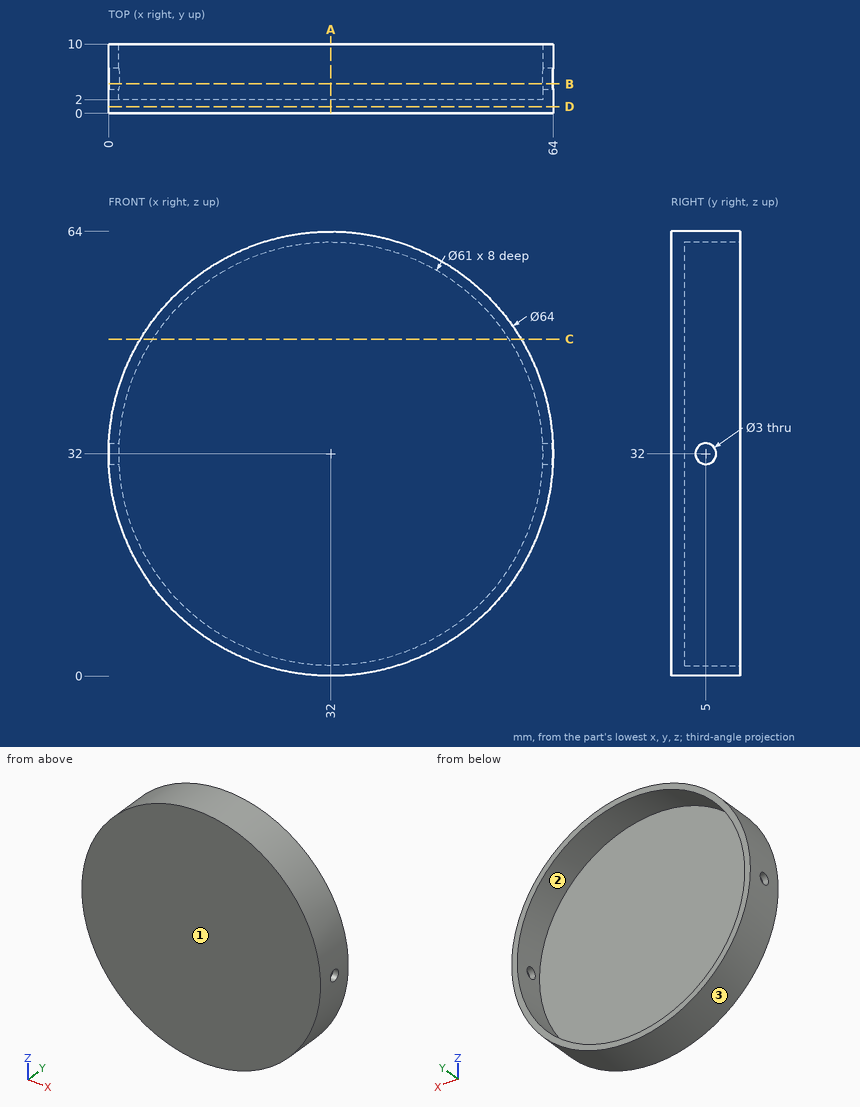
The drawing under review shows one solid part. Ordinate dimensions are in mm from its lowest x, y, z. Give positions to 0.01 mm unless a question says otherwise; leave off trailing zeros. Order: outer loops, then holes, each group sorted by start corner. A loop starts at its lowest first (then second) coordinate and runs counter-clockwise, first axis right, second up. Notation, with made-up numbers: M 4.5,28 L 26.5,28 A18 cw 26.5,52 Z; hole C 72,42 d2. An arc over 180 degrees is marked long. Answer in a Markdown table with one row per item. Add a question column.
1. Add section A-A on x = 32. State the section outline as (y, z) points, plus the area to 3 significant figures.
2. Add section B-B on y = 4.25. State the section outline as (x, z) points.
3. Add section C-C on z = 48.5. State the section outline as (x, y) points.
4. Add section D-D on y = 1. State the section outline as (x, z) points, plus the area to 3 significant figures.
5. To check wall thickness, follow line 1 along Z through (x, y) = (32, 8.5); line 2 along Y through (x, z) = (17.5, 58); line 3 along Z through (x, y) = (35, 5.75). State the ranges of each line that lie inside material, in increasing order.
6. For pin 1 Ø2 at (x, z) = (32.5, 27) entering from +Y; pin 2 Ø2.5 at (y, z) = (5, 32) entering from +X; pin 3 Ø4 at (x, y) = (29, 5.5) entering from +Z; pin 4 Ø4 at (y, z) = (6, 13.5) entering from -X, all flat-tipped, find the tip position at first contact; note any pin that passes through.
7. Mouldability with a two-part tool opening along X and no side actions: class the marked faces 1, 2 and 3 as released by +X, released by -X, zero draft, split by the parting line, or undercut.
The answers:
| question | item | result |
|---|---|---|
| 1 | outline | M 0,0 L 10,0 L 10,1.5 L 2,1.5 L 2,62.5 L 10,62.5 L 10,64 L 0,64 Z |
| 1 | area | 152 mm2 |
| 2 | outline | M 0.03,30.7 A32 ccw 63.97,30.7 L 62.47,30.7 A30.5 cw 1.53,30.7 Z; M 0.03,33.3 L 1.53,33.3 A30.5 cw 62.47,33.3 L 63.97,33.3 A32 ccw Z |
| 3 | outline | M 4.58,0 L 59.42,0 L 59.42,10 L 57.65,10 L 57.65,2 L 6.35,2 L 6.35,10 L 4.58,10 Z |
| 4 | outline | C 32,32 d64 |
| 4 | area | 3,220 mm2 |
| 5 | line 1 | 0 to 1.5, 62.5 to 64 |
| 5 | line 2 | 0 to 2 |
| 5 | line 3 | 0.14 to 1.65, 62.35 to 63.86 |
| 6 | pin 1 | y = 2 |
| 6 | pin 2 | through |
| 6 | pin 3 | z = 63.98 |
| 6 | pin 4 | x = 4.58 |
| 7 | face 1 | zero draft |
| 7 | face 2 | undercut |
| 7 | face 3 | split by the parting line |
